from build123d import *

# Parameters (mm, degrees)
F0_W     = 152.4
F0_H     = 76.2
F0_R     = 32.525
F0_R_2   = 23.5
F0_R_3   = 23
F1_DEPTH = 25.4
F2_DEPTH = 5
F3_R     = 25.527
F4_DEPTH = 6.604


with BuildPart() as f1:
    # F0 (on Top) → F1 (new body)
    with BuildSketch(Plane.XY):
        Rectangle(F0_W, F0_H)
        Circle(F0_R, mode=Mode.SUBTRACT)
        Circle(F0_R)
        Circle(F0_R_2, mode=Mode.SUBTRACT)
        Circle(F0_R_2)
        Circle(F0_R_3, mode=Mode.SUBTRACT)
        Circle(F0_R_3)
    extrude(amount=-F1_DEPTH)

    # F0 (on Top) → F2 (cut)
    with BuildSketch(Plane.XY):
        Circle(F0_R)
        Circle(F0_R_2, mode=Mode.SUBTRACT)
        Circle(F0_R_2)
        Circle(F0_R_3, mode=Mode.SUBTRACT)
    extrude(amount=-F2_DEPTH, mode=Mode.SUBTRACT)

    # F3 (on face) → F4 (cut)
    with BuildSketch(Plane(origin=(0, 0, -25.4), x_dir=(1, 0, 0), z_dir=(0, 0, -1))):
        Circle(F3_R)
    extrude(amount=-F4_DEPTH, mode=Mode.SUBTRACT)


solid = f1.part
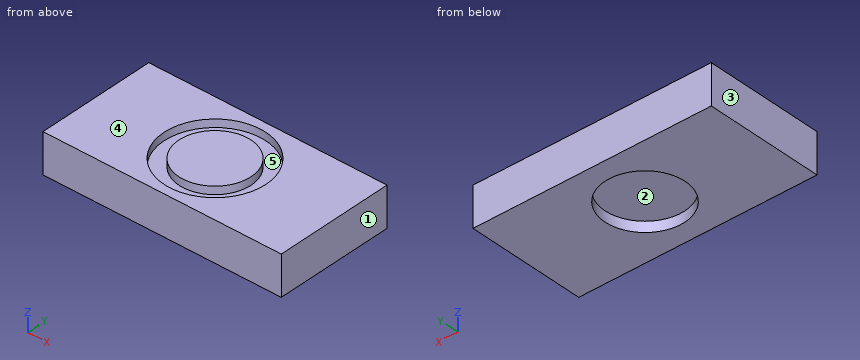
Build history of the part. All positions in model axes, mm. Face numbers are marked on the shaded views. A direction names the side the tool comes from. Coordinates: 2 decimals unless noted, no trailing zeros. Order: outer loops, then holes, each group sorted by start corner. A loop starts at its lowest first (then second) coordinate and runs counter-clockwise, first axis right, second up. Notation, with made-up numbers: (55.25, -15) - (98.25, -15) arc R32 cw to (98.25, 22) - close; hole circle Ø2 at (63.5, 54). An arc over 180 degrees is marked (long way). Put each result on its own line as item: value.
1. Saw through at C-C (y = 0). Write the cut outline in (x, z) (3 decimals), and give its area (3 significant figures).
Answer sheet:
outline: (-76.2, -25.4) - (-25.527, -25.4) - (-25.527, -18.796) - (25.527, -18.796) - (25.527, -25.4) - (76.2, -25.4) - (76.2, 0) - (32.525, 0) - (32.525, -5) - (23, -5) - (23, 0) - (-23, 0) - (-23, -5) - (-32.525, -5) - (-32.525, 0) - (-76.2, 0) - close
area: 3,440 mm^2
2. Saw through at D-D (z = -21). Write the cut outline in (x, y), and give its area (3 significant figures).
Answer sheet:
outline: (-76.2, -38.1) - (76.2, -38.1) - (76.2, 38.1) - (-76.2, 38.1) - close; hole circle Ø51.05 at (0, 0)
area: 9,570 mm^2
3. Drop flat-ended pins along their axis: P1, Ø1.5, axis at x = -14, y = -2.5, coming from the -Z side; P2, Ø8, axis at x = -47.5, y = 17.5, coming from the +Z side; P3, Ø5, axis at x = -0.5, y = 28.5, coming from the +Z side. Give the stop position or say it passes through.
Answer sheet:
P1: stops at z = -18.8
P2: stops at z = 0
P3: stops at z = -5
4. Saw through at A-A (z = -1.75). Write the cut outline in (x, y) (3 decimals).
Answer sheet:
outline: (-76.2, -38.1) - (76.2, -38.1) - (76.2, 38.1) - (-76.2, 38.1) - close; circle Ø46 at (0, 0); hole circle Ø65.05 at (0, 0)
5. Probe line 1 along Y through (x, z) = (0, -3.7) (3 decimals); line 2 along Y through (x, z) = (0, -22.25); line 3 along X through (y, z) = (-12, -2.5). List the from-to ranges inside material, lowest first. Write a range as [from, to].
Answer sheet:
line 1: y = [-38.1, -32.525], [-23, 23], [32.525, 38.1]
line 2: y = [-38.1, -25.53], [25.53, 38.1]
line 3: x = [-76.2, -30.23], [-19.62, 19.62], [30.23, 76.2]
6. Saw through at B-B (x = 0). Write the cut outline in (y, z) (3 decimals), and give its area (3 significant figures).
Answer sheet:
outline: (-38.1, -25.4) - (-25.527, -25.4) - (-25.527, -18.796) - (25.527, -18.796) - (25.527, -25.4) - (38.1, -25.4) - (38.1, 0) - (32.525, 0) - (32.525, -5) - (23, -5) - (23, 0) - (-23, 0) - (-23, -5) - (-32.525, -5) - (-32.525, 0) - (-38.1, 0) - close
area: 1,500 mm^2
7. Tool access for the marked faces 1 and 2: list every direction of +Z, -Z, +X, -X, +Y, -Y with a clear straight run to the whole face (end or side of a thin tool).
Answer sheet:
face 1: +Z, -Z, +X, +Y, -Y
face 2: -Z
8. Pull direction X, two halves, no side cores. Call the marked faces 3, 4 and 5: pulls with the +X half, pulls with the -X half, needs draft (parallel to the pull), parting line crosses it, or undercut.
Answer sheet:
face 3: pulls with the -X half
face 4: needs draft
face 5: undercut
